from build123d import *

# Parameters (mm, degrees)
SKETCH1_W           = 330.2
SKETCH1_H           = 438.15
SKETCH1_R           = 14.2875
SKETCH1_R_2         = 11.176
BOSS_EXTRUDE1_DEPTH = 4.7625
SKETCH2_R           = 14.2875
CUT_EXTRUDE1_DEPTH  = 4.7625
SKETCH3_R           = 14.2875
CUT_EXTRUDE2_DEPTH  = 4.7625
SKETCH4_R           = 2.667
CUT_EXTRUDE3_DEPTH  = 549.662140034


with BuildPart() as part:
    # Sketch1 → Boss-Extrude1 (new body)
    with BuildSketch(Plane.XY):
        with Locations((165.1, -219.075)):
            Rectangle(SKETCH1_W, SKETCH1_H)
        with Locations(Location((270.114426387, -191.844382727, 0), (0, 0, 180))):
            Circle(SKETCH1_R, mode=Mode.SUBTRACT)
        with Locations(Location((101.925695163, -306.813385495, 0), (0, 0, 180))):
            Circle(SKETCH1_R_2, mode=Mode.SUBTRACT)
        with Locations(Location((64.374426387, -313.256382727, 0), (0, 0, 180))):
            Circle(SKETCH1_R_2, mode=Mode.SUBTRACT)
    extrude(amount=BOSS_EXTRUDE1_DEPTH)

    # Sketch2 → Cut-Extrude1 (cut)
    with BuildSketch(Plane.XY.offset(4.7625)):
        with Locations((66.914426387, -355.904507537)):
            Circle(SKETCH2_R)
    extrude(amount=-CUT_EXTRUDE1_DEPTH, mode=Mode.SUBTRACT)

    # Sketch3 → Cut-Extrude2 (cut)
    with BuildSketch(Plane.XY.offset(4.7625)):
        with Locations((117.714426387, -362.254507537)):
            Circle(SKETCH3_R)
        with Locations((168.514426387, -368.604507537)):
            Circle(SKETCH3_R)
        with Locations((219.314426387, -374.954507537)):
            Circle(SKETCH3_R)
        with Locations((270.114426387, -381.304507537)):
            Circle(SKETCH3_R)
    extrude(amount=-CUT_EXTRUDE2_DEPTH, mode=Mode.SUBTRACT)

    # Sketch4 → Cut-Extrude3 (cut, through all)
    with BuildSketch(Plane(origin=(0, 0, 0), x_dir=(-1, 0, 0), z_dir=(0, 0, -1))):
        with Locations((-12.7, -425.45)):
            Circle(SKETCH4_R)
        with Locations((-12.7, -412.75)):
            Circle(SKETCH4_R)
        with Locations((-12.7, -400.05)):
            Circle(SKETCH4_R)
        with Locations((-12.7, -387.35)):
            Circle(SKETCH4_R)
        with Locations((-12.7, -374.65)):
            Circle(SKETCH4_R)
        with Locations((-12.7, -361.95)):
            Circle(SKETCH4_R)
        with Locations((-12.7, -349.25)):
            Circle(SKETCH4_R)
        with Locations((-12.7, -336.55)):
            Circle(SKETCH4_R)
        with Locations((-12.7, -44.45)):
            Circle(SKETCH4_R)
        with Locations((-12.7, -31.75)):
            Circle(SKETCH4_R)
        with Locations((-12.7, -19.05)):
            Circle(SKETCH4_R)
        with Locations((-317.5, -361.95)):
            Circle(SKETCH4_R)
        with Locations((-317.5, -349.25)):
            Circle(SKETCH4_R)
        with Locations((-317.5, -336.55)):
            Circle(SKETCH4_R)
        with Locations((-317.5, -400.05)):
            Circle(SKETCH4_R)
        with Locations((-317.5, -412.75)):
            Circle(SKETCH4_R)
        with Locations((-317.5, -425.45)):
            Circle(SKETCH4_R)
        with Locations((-317.5, -44.45)):
            Circle(SKETCH4_R)
        with Locations((-317.5, -31.75)):
            Circle(SKETCH4_R)
        with Locations((-317.5, -19.05)):
            Circle(SKETCH4_R)
        with Locations((-25.4, -425.45)):
            Circle(SKETCH4_R)
        with Locations((-38.1, -425.45)):
            Circle(SKETCH4_R)
        with Locations((-50.8, -425.45)):
            Circle(SKETCH4_R)
        with Locations((-63.5, -425.45)):
            Circle(SKETCH4_R)
        with Locations((-76.2, -425.45)):
            Circle(SKETCH4_R)
        with Locations((-88.9, -425.45)):
            Circle(SKETCH4_R)
        with Locations((-101.6, -425.45)):
            Circle(SKETCH4_R)
        with Locations((-114.3, -425.45)):
            Circle(SKETCH4_R)
        with Locations((-127, -425.45)):
            Circle(SKETCH4_R)
        with Locations((-139.7, -425.45)):
            Circle(SKETCH4_R)
        with Locations((-152.4, -425.45)):
            Circle(SKETCH4_R)
        with Locations((-165.1, -425.45)):
            Circle(SKETCH4_R)
        with Locations((-177.8, -425.45)):
            Circle(SKETCH4_R)
        with Locations((-190.5, -425.45)):
            Circle(SKETCH4_R)
        with Locations((-203.2, -425.45)):
            Circle(SKETCH4_R)
        with Locations((-215.9, -425.45)):
            Circle(SKETCH4_R)
        with Locations((-228.6, -425.45)):
            Circle(SKETCH4_R)
        with Locations((-241.3, -425.45)):
            Circle(SKETCH4_R)
        with Locations((-254, -425.45)):
            Circle(SKETCH4_R)
        with Locations((-266.7, -425.45)):
            Circle(SKETCH4_R)
        with Locations((-279.4, -425.45)):
            Circle(SKETCH4_R)
        with Locations((-292.1, -425.45)):
            Circle(SKETCH4_R)
        with Locations((-304.8, -425.45)):
            Circle(SKETCH4_R)
    extrude(amount=-CUT_EXTRUDE3_DEPTH, mode=Mode.SUBTRACT)


solid = part.part
Read the model definition and answer for the solid it produces. Units are mm, in the model's axes. Round coordinates to 2 decimals unless told otherwise and drop trailing zeros. One line per question, with ' | ' between items. Start each with the question number.
Q1. A flat-ended cylindrical pin translates along its axis: pin 1 (3 mm diameter, centred on x = 12.7, y = -374.65, fed in from -Z). Find the tip coordinate at first contact, or state that the pin passes through.
Q2. Find the intervals of material crossed by L1, parallel to X at y = -411.5, z = 4.4; L2, parallel to Y at x = 169, z = 1.6; L3, parallel to Y at x = 78, z = 4.1, in increasing order.
Q3. For a pull along Y with two mould halves and no side action, classify faces 1 (the flat face through (163, -216, 0)), 2 (the cylindrical face through (281.45, -183.15, 2.35)) as +Y half, -Y half, draft (parallel to the pull), parting line (faces both ways), or undercut.
Q4. Section A-A on z = 2.5 is taken. Count the separate pieces of the cut face and the enclosed holes in it, plus the area to 3 significant figures.
Established:
1) pin 1: through
2) L1: 0 to 10.34, 15.06 to 315.14, 319.86 to 330.2 | L2: -438.15 to -382.88, -354.33 to 0 | L3: -438.15 to -427.42, -423.48 to -364.92, -346.89 to 0
3) face 1: draft | face 2: undercut
4) separate pieces: 1 | enclosed holes: 51 | area: 139,000 mm²
